Could you check a few things on this model? Use its own coordinates, in mm. Face numbers are marked on the shaded views. A direction names the side the tool comes from. Coordinates: 2 decimals unless noted, no trailing zeros. Write each loop counter-clockwise with the first axis right and the second up, starting at its lowest first coordinate (ties: lowest second). Pieces come first, ordered by that corner, then holes. Notation, with made-up numbers: M 63,57 L 102,57 A15 cw 102,84 Z; hole C 51.5,-24 d5. An arc over 180 degrees is marked long. Answer as CSV lines item,"result". Start each with the question number.
Item 1: Suppose I cut it at D-D, the plane x = -2.75. Write out the boundary of the cut face in (y, z), and give its area (3 significant figures).
Item 2: Suppose I cut it at A-A, the plane y = -3.5. Write out the boundary of the cut face in (x, z), and give its area (3 significant figures).
Item 3: I'm going to push flat-ended pins straight in: P1, Ø1.5, axis at x = -3, y = -3.5, coming from the -Z side; P2, Ø0.9, axis at y = -3.5, z = -0.5, coming from the -X side; P3, Ø1.5, axis at y = -4, z = 0.5, coming from the +X side. Where does each tip first touch, or does it pass through?
Item 4: On a 3-axis mill with a long thin cutter (end or side, diameter ignored), from which of +Z, -Z, +X, -X, +Y, -Y can I reach the whole of each face in a straight line? I mean the marked faces 1, 2 and 3. Say none if no direction works.
Item 5: If I drill on line 1 along Z through (x, y) = (0, -1.4); line 2 along Y through (x, z) = (0.85, 0); line 3 along Y through (x, z) = (-2, -1), over which ranges is the centre line in solid material (lowest first)? Write a range as [from, to].
Item 6: Suppose I cut it at B-B, the plane z = 0.25. Write out the boundary of the cut face in (x, y).
Item 7: We'd pull the mould along X, two halves only. Please class the marked faces 4, 5 and 6: +X half, -X half, draft (parallel to the pull), parting line (faces both ways), or undercut.
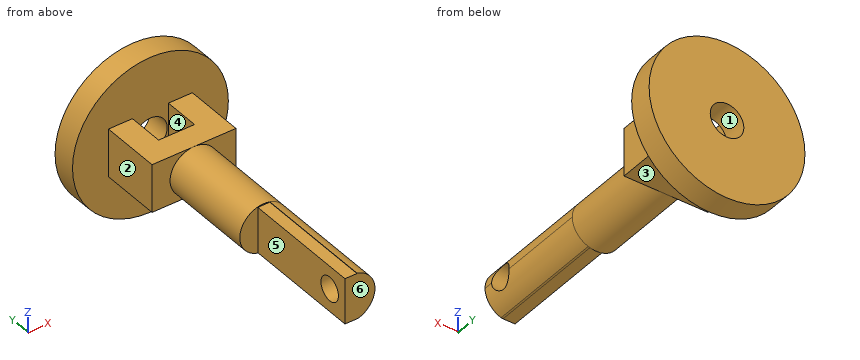
```python
from build123d import *

# Parameters (mm, degrees)
F0_R      = 6.5
F0_W      = 2
F0_H      = 4
F0_R_2    = 1.4
F1_DEPTH  = 2
F2_DEPTH  = 5
F3_W      = 7
F3_H      = 4
F4_DEPTH  = 2
F5_R      = 2
F6_DEPTH  = 8
F7_W      = 1
F7_H      = 3.8
F8_DEPTH  = 10
F9_R      = 1
F10_DEPTH = 3.46
F11_DEPTH = 10
F12_DEPTH = 2.95


with BuildPart() as f1:
    # F0 (on Front) → F1 (new body)
    with BuildSketch(Plane.XZ):
        Circle(F0_R)
        with Locations((-2.5, 0)):
            Rectangle(F0_W, F0_H, mode=Mode.SUBTRACT)
        Circle(F0_R_2, mode=Mode.SUBTRACT)
        with Locations((2.5, 0)):
            Rectangle(F0_W, F0_H, mode=Mode.SUBTRACT)
    extrude(amount=F1_DEPTH)

    # F0 (on Front) → F2 (join)
    with BuildSketch(Plane.XZ):
        with Locations((-2.5, 0)):
            Rectangle(F0_W, F0_H)
        with Locations((2.5, 0)):
            Rectangle(F0_W, F0_H)
    extrude(amount=F2_DEPTH)

    # F3 (on face) → F4 (join)
    with BuildSketch(Plane.XZ.offset(5)):
        Rectangle(F3_W, F3_H)
    extrude(amount=F4_DEPTH)

    # F5 (on face) → F6 (join)
    with BuildSketch(Plane.XZ.offset(7)):
        Circle(F5_R)
    extrude(amount=F6_DEPTH)

    # F7 (on face) → F8 (join)
    with BuildSketch(Plane.XZ.offset(15)):
        Rectangle(F7_W, F7_H)
    extrude(amount=F8_DEPTH)

    # F9 (on face) → F10 (cut)
    with BuildSketch(Plane(origin=(-0.5, 0, 0), x_dir=(0, -1, 0), z_dir=(-1, 0, 0))):
        with Locations((23.2482682914, 0)):
            Circle(F9_R)
    extrude(amount=-F10_DEPTH, mode=Mode.SUBTRACT)

    # F7 (on face) → F11 (join)
    with BuildSketch(Plane.XZ.offset(15)):
        with BuildLine():
            Line((0.5, 1.9), (0.5, -1.9))
            Line((0.5, -1.9), (0.667421366, -1.8853510867))
            ThreePointArc((0.667421366, -1.8853510867), (1.633224224, -1.1543736977), (2, 0))
            ThreePointArc((2, 0), (1.5811388301, 1.2247448714), (0.5, 1.9364916731))
            Line((0.5, 1.9364916731), (0.5, 1.9))
        make_face()
    extrude(amount=F11_DEPTH)

    # F12 (cut): a face of the model
    f12_faces = [f1.faces().sort_by_distance(p)[0] for p in [
        (0.5, -23.2482682914, 0),
    ]]
    extrude(f12_faces, amount=-F12_DEPTH, mode=Mode.SUBTRACT)


solid = f1.part
```
Ans:
1,outline,"M -7,-2 L -2,-2 L -2,-5.89 L 0,-5.89 L 0,5.89 L -2,5.89 L -2,2 L -7,2 Z"
1,area,"43.6 mm^2"
2,outline,"M -3.5,-2 L -1.5,-2 L -1.5,2 L -3.5,2 Z; M 1.5,-2 L 3.5,-2 L 3.5,2 L 1.5,2 Z"
2,area,"16.0 mm^2"
3,P1,"stops at z = -2"
3,P2,"stops at x = -3.5"
3,P3,"stops at x = 3.5"
4,face 1,"+Y"
4,face 2,"+Z, -Z, -X, -Y"
4,face 3,"-Z, +X, -X, -Y"
5,line 1,"z = [-6.5, -1.4], [1.4, 6.5]"
5,line 2,"y = [-25, -24.25], [-22.25, -5]"
5,line 3,"y = [-7, 0]"
6,outline,"M -6.5,-2 L -3.5,-2 L -3.5,-7 L -1.98,-7 L -1.98,-15 L -0.5,-15 L -0.5,-22.28 L 1.98,-22.28 L 1.98,-7 L 3.5,-7 L 3.5,-2 L 6.5,-2 L 6.5,0 L 1.38,0 L 1.38,-2 L 1.5,-2 L 1.5,-5 L -1.5,-5 L -1.5,-2 L -1.38,-2 L -1.38,0 L -6.5,0 Z; M -0.5,-25 L 1.98,-25 L 1.98,-24.22 L -0.5,-24.22 Z"
7,face 4,"undercut"
7,face 5,"-X half"
7,face 6,"draft"
